Can you work these out from the drawing? Everything is in mm from the part's minimum corner. A direction names the side the tool comes from. Round coordinates to 2 decimals unless told otherwise and drop trailing zeros. Loops run counter-clockwise (first coordinate to the right, second up) from the corner with the lowest first, then second, coordinate; pieces in that order, holes last. Notation, with made-up numbers: M 32,59.5 L 85,59.5 A23 ccw 85,69.5 Z; hole C 80,-24.5 d11. An arc over 180 degrees is marked long. Answer in a Markdown table with one row per item.
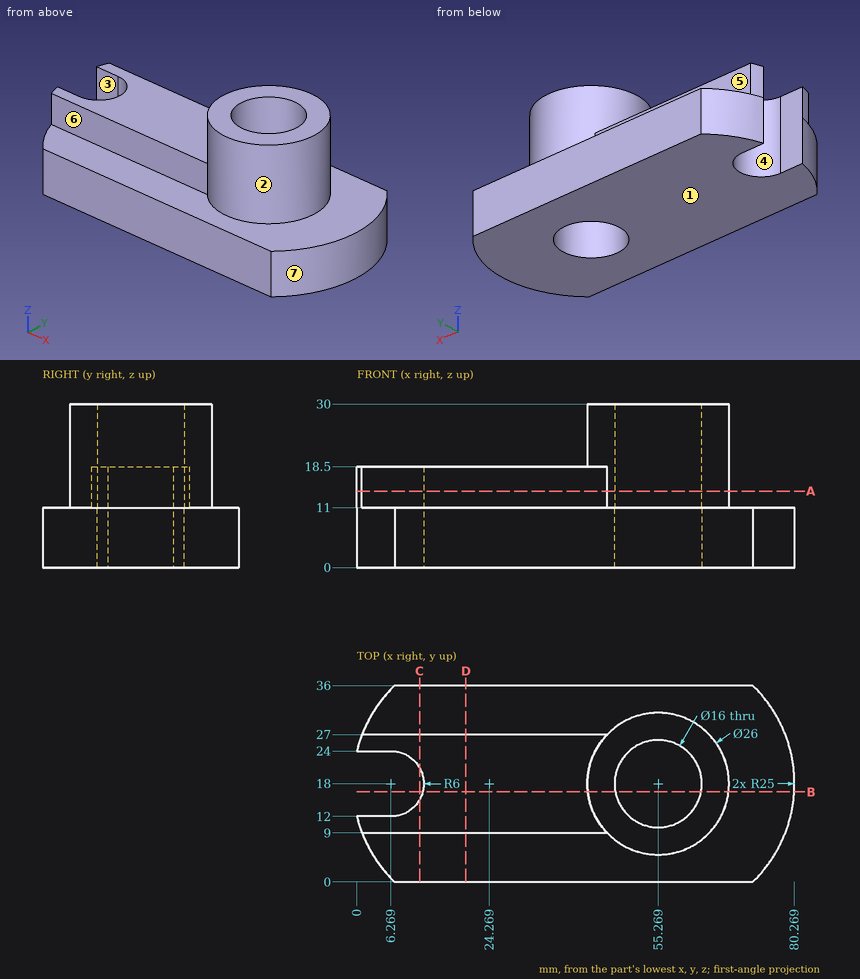
1) Will these pins go through, and if not, where does the flat tip stop? P1, Ø11, axis at x = 31, y = 27, coming from the +Z side; P2, Ø3, axis at x = 2.5, z = 5, coming from the -Y side (1 decimal); P3, Ø6, axis at y = 9, z = 22.5, coming from the +X side; P4, Ø3, axis at x = 61, y = 16, coming from the +Z side.
Computed:
| item | result |
|---|---|
| P1 | stops at z = 18.5 |
| P2 | stops at y = 3.4 |
| P3 | stops at x = 66.8 |
| P4 | passes through |
2) I want a section at D-D, the plane x = 20. Please give me the cut outline in (y, z).
Computed:
| item | result |
|---|---|
| outline | M 0,0 L 36,0 L 36,11 L 27,11 L 27,18.5 L 9,18.5 L 9,11 L 0,11 Z |
3) I want a section at C-C, the plane x = 11.5. Please give me the cut outline in (y, z), plus the area to 3 significant figures.
Computed:
| item | result |
|---|---|
| outline | M 0,0 L 15.06,0 L 15.06,18.5 L 9,18.5 L 9,11 L 0,11 Z; M 20.94,0 L 36,0 L 36,11 L 27,11 L 27,18.5 L 20.94,18.5 Z |
| area | 422 mm² |
4) I need wall thicknesses on line 1 (Z direction, x = 30, y = 13.5); line 2 (X direction, y = 11.5, z = 6) (1 decimal); line 3 (Z direction, x = 25, y = 27.5). Which ranges of each line are inside material? Lowest first, please.
Computed:
| item | result |
|---|---|
| line 1 | z = 0 to 18.5 |
| line 2 | x = 0.1 to 50.6, 59.9 to 79.4 |
| line 3 | z = 0 to 11 |
5) Which directions (+Z, -Z, +X, -X, +Y, -Y) give clear straight access to the entire face, cutting with the end or side of a thin tool? Please do the marked faces 1, 2 and 3.
Computed:
| item | result |
|---|---|
| face 1 | -Z, +X, -X, +Y, -Y |
| face 2 | +Z |
| face 3 | +Z, -Z, -X |
6) I want a section at B-B, the plane y = 16.5. Please give me the cut outline in (x, z), plus the area to 3 significant figures.
Computed:
| item | result |
|---|---|
| outline | M 12.08,0 L 47.41,0 L 47.41,30 L 42.36,30 L 42.36,18.5 L 12.08,18.5 Z; M 63.13,0 L 80.22,0 L 80.22,11 L 68.18,11 L 68.18,30 L 63.13,30 Z |
| area | 996 mm² |
7) If we mould it in two halves opening along Y, with no side actions, what happens to the marked faces 4, 5, 6 and 7? For each: released by +Y, released by -Y, zero draft, split by the parting line, or undercut.
Computed:
| item | result |
|---|---|
| face 4 | undercut |
| face 5 | released by +Y |
| face 6 | released by -Y |
| face 7 | split by the parting line |
8) I want a section at A-A, the plane z = 14. Please give me the cut outline in (x, y) (1 decimal).
Computed:
| item | result |
|---|---|
| outline | M 0,12 A25 ccw 0.9,9 L 45.9,9 A13 ccw long 45.9,27 L 0.9,27 A25 ccw 0,24 L 6.3,24 A6 cw 6.3,12 Z; hole C 55.3,18 d16 |
